from build123d import *

# Parameters (mm, degrees)
F1_DEPTH       = 76.2
F3_D           = 38.1
F3_DEPTH       = 38.1
F3_CBORE_D     = 50.8
F3_CBORE_DEPTH = 12.7
F3_TIP         = 11.4463947925
F4_D           = 41.148
F4_DEPTH       = 76.2
F4_CBORE_D     = 50.8
F4_CBORE_DEPTH = 12.7
F4_TIP         = 12.3621063759


with BuildPart() as f1:
    # F0 (on Right) → F1 (new body)
    with BuildSketch(Plane.YZ):
        with BuildLine():
            ThreePointArc((-0.3445927945, 76.0475993156), (-37.9475988448, 113.6506053659), (-75.5506048951, 76.0475993156))
            Line((-75.5506048951, 76.0475993156), (-0.3445927945, 76.0475993156))
        make_face()
        Polygon((-75.8951976895, 76.0475993156), (-75.8951976895, 0), (0, 0), (0, 76.0475993156), (-0.3445927945, 76.0475993156), (-75.5506048951, 76.0475993156), align=None)
        Polygon((0, 0), (-75.8951976895, 0), (-75.8951976895, -28.1940009445), (103.6320030689, -28.1940009445), (103.6320030689, 0), align=None)
    extrude(amount=F1_DEPTH)

    # F3
    with Locations(Plane.XY):
        with Locations((38.2905006409, 65.7788068056)):
            CounterBoreHole(F3_D / 2, F3_CBORE_D / 2, F3_CBORE_DEPTH, depth=F3_DEPTH)
            with Locations((0, 0, -(F3_DEPTH + F3_TIP / 2))):  # 118° drill point
                Cone(0, F3_D / 2, F3_TIP, mode=Mode.SUBTRACT)

    # F4
    with Locations(Plane(origin=(0, 0, 0), x_dir=(0, 1, 0), z_dir=(-1, 0, 0))):
        with Locations((-37.9475988448, -76.0475993156)):
            CounterBoreHole(F4_D / 2, F4_CBORE_D / 2, F4_CBORE_DEPTH, depth=F4_DEPTH)
            with Locations((0, 0, -(F4_DEPTH + F4_TIP / 2))):  # 118° drill point
                Cone(0, F4_D / 2, F4_TIP, mode=Mode.SUBTRACT)


solid = f1.part
Source: CAD feature listing. Evaluate the final solid. Frame: model axes, mm. A direction names the side the tool comes from. Coordinates: 2 decimals unless noted, no trailing zeros. Loops run counter-clockwise (first coordinate to the right, second up) from the corner with the lowest first, then second, coordinate; pieces in that order, holes last. Notation, with made-up numbers: (-9, 85) - (14, 85) arc R21 cw to (14, 94) - close; hole circle Ø4 at (14.25, 11). An arc over 180 degrees is marked (long way). Return JSON: item names as keys, results as strings.
Q1. Mould query, pull axis Z, two halves, no side actions, for faces 5 (the flat face through (38, 13, -28.194)), 6 (the cylindrical face through (44.89, -35.27, 55.65)), 7 (the flat face through (38, -75.895, 25)). Classes: released by +Z, released by -Z, zero draft, split by the parting line, or undercut.
Results:
{"face 5": "released by -Z", "face 6": "undercut", "face 7": "zero draft"}
Q2. Section C-C, the plane z = 87. Return loops of the section in (x, y), plus the area to 3 significant figures.
Results:
{"outline": "(0, -73.92) - (76.2, -73.92) - (76.2, -55.36) - (12.7, -55.36) - (12.7, -60.86) - (0, -60.86) - close; (0, -15.03) - (12.7, -15.03) - (12.7, -20.53) - (76.2, -20.53) - (76.2, -1.97) - (0, -1.97) - close", "area": "2,690 mm2"}
Q3. Section B-B, the plane y = 53. Return loops of the section in (x, z).
Results:
{"outline": "(0, -28.19) - (24.16, -28.19) - (24.16, -12.7) - (16.34, -12.7) - (16.34, 0) - (0, 0) - close; (52.42, -28.19) - (76.2, -28.19) - (76.2, 0) - (60.24, 0) - (60.24, -12.7) - (52.42, -12.7) - close"}
Q4. Material intervals for line 1 along Y through (x, z) = (14, 76); line 2 along Y through (x, z) = (48, 38); line 3 along Z through (x, y) = (53, 38), sorted ascending.
Results:
{"line 1": "-75.9 to -58.52, -17.37 to 0", "line 2": "-75.9 to 0", "line 3": "-28.19 to 0"}
Q5. Access query for faces 1 (the flat face through (38, 0, 37)), 2 (the flat face through (42, 85, -12.7)), 3 (the cylindrical face through (6.261, -58.104, 91.503)), 4 (the flat face through (76.2, -7, 28)). Directions: +Z, -Z, +X, -X, +Y, -Y. A direction counts if a zero-diameter tool reaches every point of the face in a straight line with its end or side. Return the directions, or none.
Results:
{"face 1": "+Z, +X, -X, +Y", "face 2": "+Z", "face 3": "-X", "face 4": "+Z, -Z, +X, +Y, -Y"}
Q6. Section A-A, the plane x = 8.5. Return loops of the section in (y, z), plus the area to 3 significant figures.
Results:
{"outline": "(-75.9, -28.19) - (103.63, -28.19) - (103.63, 0) - (0, 0) - (0, 76.05) - (-0.34, 76.05) arc R37.6 ccw to (-75.55, 76.05) - (-75.9, 76.05) - close; hole circle Ø50.8 at (-37.95, 76.05)", "area": "11,000 mm2"}
Q7. Section D-D, the plane x = 33. Return loops of the section in (y, z), plus the area to 3 significant figures.
Results:
{"outline": "(-75.9, -28.19) - (47.48, -28.19) - (47.48, -12.7) - (40.94, -12.7) - (40.94, 0) - (0, 0) - (0, 76.05) - (-0.34, 76.05) arc R37.6 ccw to (-75.55, 76.05) - (-75.9, 76.05) - close; (84.08, -28.19) - (103.63, -28.19) - (103.63, 0) - (90.62, 0) - (90.62, -12.7) - (84.08, -12.7) - close; hole circle Ø41.15 at (-37.95, 76.05)", "area": "10,500 mm2"}
